Build history of the part. All positions in model axes, mm. A direction names the side the tool comes from. Give positions to 0.01 mm unless a question says otherwise; leave off trailing zeros. Order: outer loops, then holes, each group sorted by start corner. A loop starts at its lowest first (then second) coordinate and runs counter-clockwise, first axis right, second up. Notation, with made-up numbers: (28, 69.25) -> (82, 69.25) arc R35 cw to (82, 101.25) -> close; hole circle Ø4 at (40.5, -35.75). An arc over 180 degrees is marked (long way). One line per question, with ' | ' between items. Start each with the question number.
(1) Pull direction Z, two halves, no side cores. Call faces 3 (the face through (15.466, 0.176, 71.004)), 4 (the face through (-1.256, -15.28, 6.846)), 5 (the face through (0, -15, 74)): +Z half, -Z half, draft (parallel to the pull), parting line (faces both ways), or undercut.
(2) Cut at D-D (z = 75). Give the cut face in (x, y).
(3) Cut at C-C (x = 8). Give the cut face in (y, z).
(4) Cut at A-A (z = 127). Give the cut face in (x, y), then the cut area to 3 significant figures.
(5) Which spindle directions (+Z, -Z, +X, -X, +Y, -Y) get a long thin tool onto all of the face, cutting with end or side? Do faces 1 (the face through (0, 15.945, 74)), 2 (the face through (15, -7, 74)). Say none if no direction does.
(6) Drill centre lines: L1, parallel to Y at x = 11.5, z = 45; L2, parallel to Y at x = -15.35, z = 75. Where is each one in solid material? Low to high. Write a range as from..to.
(7) Cut at B-B (y = 0). Give the cut face in (x, z).
from build123d import *

# Parameters (mm, degrees)
ESBO_O1_W                = 31.890446896
ESBO_O1_H                = 31.890446896
ESBO_O1_W_2              = 30
ESBO_O1_H_2              = 30
RESSALTO_EXTRUS_O1_DEPTH = 149.11688245
CORTE_EXTRUS_O1_DEPTH    = 154.320238017
ESBO_O4_R                = 4
CORTE_EXTRUS_O2_DEPTH    = 32


with BuildPart() as part:
    # Esboço1 → Ressalto-extrusão1 (new body)
    with BuildSketch(Plane.XY):
        Rectangle(ESBO_O1_W, ESBO_O1_H)
        Rectangle(ESBO_O1_W_2, ESBO_O1_H_2, mode=Mode.SUBTRACT)
    extrude(amount=RESSALTO_EXTRUS_O1_DEPTH)

    # Esboço3 → Corte-extrusão1 (cut, symmetric)
    with BuildSketch(Plane(origin=(0, 15.945223448, 0), x_dir=(1, 0, 0), z_dir=(0, 1, 0))):
        Polygon((-15.945223448, -12.692594834), (15.945223448, 0), (-15.945223448, 0), align=None)
    corte_extrus_o1 = extrude(amount=CORTE_EXTRUS_O1_DEPTH, both=True, mode=Mode.SUBTRACT)

    # Espelhar5: Corte-extrusão1 across plane
    add(corte_extrus_o1.mirror(Plane(origin=(0, 0, 74.558441225), x_dir=(1, 0, 0), z_dir=(0, 0, -1))), mode=Mode.SUBTRACT)

    # Esboço4 → Corte-extrusão2 (cut)
    with BuildSketch(Plane.ZY.offset(15.945223448)):
        with Locations((75, 0)):
            Circle(ESBO_O4_R)
    extrude(amount=-CORTE_EXTRUS_O2_DEPTH, mode=Mode.SUBTRACT)


solid = part.part
Result set:
1) face 3: undercut | face 4: -Z half | face 5: draft
2) outline: (-15.95, -15.95) -> (15.95, -15.95) -> (15.95, -4) -> (15, -4) -> (15, -15) -> (-15, -15) -> (-15, -4) -> (-15.95, -4) -> close; (-15.95, 4) -> (-15, 4) -> (-15, 15) -> (15, 15) -> (15, 4) -> (15.95, 4) -> (15.95, 15.95) -> (-15.95, 15.95) -> close
3) outline: (-15.95, 3.16) -> (-15, 3.16) -> (-15, 145.95) -> (-15.95, 145.95) -> close; (15, 3.16) -> (15.95, 3.16) -> (15.95, 145.95) -> (15, 145.95) -> close
4) outline: (-15.95, -15.95) -> (15.95, -15.95) -> (15.95, 15.95) -> (-15.95, 15.95) -> close; hole (-15, -15) -> (15, -15) -> (15, 15) -> (-15, 15) -> close | area: 117 mm2
5) face 1: +Z, -Z, +X, -X, +Y | face 2: +Z, -Z
6) L1: y = -15.95..-15, 15..15.95 | L2: y = -15.95..-4, 4..15.95
7) outline: (-15.95, 12.69) -> (-15, 12.32) -> (-15, 71) -> (-15.95, 71) -> close; (-15.95, 79) -> (-15, 79) -> (-15, 136.8) -> (-15.95, 136.42) -> close; (15, 0.38) -> (15.95, 0) -> (15.95, 71) -> (15, 71) -> close; (15, 79) -> (15.95, 79) -> (15.95, 149.12) -> (15, 148.74) -> close
